from build123d import *

# Parameters (mm, degrees)
SKETCH1_R           = 8.89
SKETCH1_R_2         = 6.477
BOSS_EXTRUDE1_DEPTH = 63.5
SKETCH2_R           = 8.89
SKETCH2_R_2         = 6.477
BOSS_EXTRUDE2_DEPTH = 31.75
SKETCH4_R           = 6.477
CUT_EXTRUDE1_DEPTH  = 64.5000001
SKETCH5_R           = 6.477
CUT_EXTRUDE2_DEPTH  = 64.5000001


with BuildPart() as part:
    # Sketch1 → Boss-Extrude1 (new body)
    with BuildSketch(Plane.XY):
        Circle(SKETCH1_R)
        Circle(SKETCH1_R_2, mode=Mode.SUBTRACT)
    extrude(amount=BOSS_EXTRUDE1_DEPTH)

    # Sketch2 → Boss-Extrude2 (add, symmetric)
    with BuildSketch(Plane(origin=(0, 0, 0), x_dir=(0, 0, -1), z_dir=(1, 0, 0))):
        with Locations((-31.75, 0)):
            Circle(SKETCH2_R)
        with Locations((-31.75, 0)):
            Circle(SKETCH2_R_2, mode=Mode.SUBTRACT)
    extrude(amount=BOSS_EXTRUDE2_DEPTH, both=True)

    # Sketch4 → Cut-Extrude1 (cut, through all)
    with BuildSketch(Plane(origin=(0, 0, 0), x_dir=(-1, 0, 0), z_dir=(0, 0, -1))):
        Circle(SKETCH4_R)
    extrude(amount=-CUT_EXTRUDE1_DEPTH, mode=Mode.SUBTRACT)

    # Sketch5 → Cut-Extrude2 (cut, through all)
    with BuildSketch(Plane(origin=(31.75, 0, 0), x_dir=(0, 0, -1), z_dir=(1, 0, 0))):
        with Locations((-31.75, 0)):
            Circle(SKETCH5_R)
    extrude(amount=-CUT_EXTRUDE2_DEPTH, mode=Mode.SUBTRACT)


solid = part.part
Check sheet for the modelled part. Datum: model origin and axes. Units: mm. A direction names the side the tool comes from. Round coordinates to 2 decimals unless told otherwise and drop trailing zeros. Loops run counter-clockwise (first coordinate to the right, second up) from the corner with the lowest first, then second, coordinate; pieces in that order, holes last.
1. Sectioned sample at B-B on z = 27. Record the boundary of the cut face in (x, y), and give its area (3 significant figures).
2. Set-up check for faces 3 (the cylindrical face through (-19.18, 2.67, 23.27)), 4 (the cylindrical face through (8.212, -3.405, 12.125)), 5 (the cylindrical face through (8.48, 2.67, 50.93)): record each of +Z, -Z, +X, -X, +Y, -Y from which the full face is reachable in a straight line by a thin tool's end or side.
3. Sectioned sample at A-A on y = 0. Record the boundary of the cut face in (x, z), and give its area (3 significant figures).
4. Mould release check, pull along Y, two halves, no side actions. Record for faces 1 (the cylindrical face through (19.625, -3.405, 23.538)), 2 (the flat face through (31.75, -7, 31)): released by +Y, released by -Y, zero draft, split by the parting line, or undercut.
5. Gauge pin test, flat ends, axial feed: pin 1 Ø8 at (x, z) = (-22.5, 47.5) entering from -Y; pin 2 Ø8 at (x, z) = (-20.5, 36) entering from +Y; pin 3 Ø1 at (y, z) = (-2.5, 15) entering from +X; pin 4 Ø1.5 at (x, z) = (6.5, 36) entering from +Y. Record the tip position at first contact, or that the pin passes through.
6. Scan lines: probe 1 along Y at (x, z) = (-6, 31.75); probe 2 along Z at (x, y) = (12, 0); probe 3 along X at (y, z) = (-0.75, 4). Record each from-to range of solid material in increasing order.
7. Sectioned sample at D-D on y = -3.25. Record the boundary of the cut face in (x, z), and give its area (3 significant figures).
8. Sectioned sample at C-C on x = -20. Record the boundary of the cut face in (y, z).
Recorded:
1. outline: (-31.75, -7.51) - (-4.75, -7.51) arc R8.89 ccw to (4.75, -7.51) - (31.75, -7.51) - (31.75, -4.4) - (4.75, -4.4) arc R6.48 cw to (-4.75, -4.4) - (-31.75, -4.4) - close; (-31.75, 4.4) - (-4.75, 4.4) arc R6.48 cw to (4.75, 4.4) - (31.75, 4.4) - (31.75, 7.51) - (4.75, 7.51) arc R8.89 ccw to (-4.75, 7.51) - (-31.75, 7.51) - close
1. area: 386 mm2
2. face 3: -X
2. face 4: -Z
2. face 5: +Z
3. outline: (-31.75, 22.86) - (-8.89, 22.86) - (-8.89, 0) - (-6.48, 0) - (-6.48, 25.27) - (-31.75, 25.27) - close; (-31.75, 38.23) - (-6.48, 38.23) - (-6.48, 63.5) - (-8.89, 63.5) - (-8.89, 40.64) - (-31.75, 40.64) - close; (6.48, 0) - (8.89, 0) - (8.89, 22.86) - (31.75, 22.86) - (31.75, 25.27) - (6.48, 25.27) - close; (6.48, 38.23) - (31.75, 38.23) - (31.75, 40.64) - (8.89, 40.64) - (8.89, 63.5) - (6.48, 63.5) - close
3. area: 465 mm2
4. face 1: split by the parting line
4. face 2: zero draft
5. pin 1: passes through
5. pin 2: stops at y = 8.89
5. pin 3: stops at x = 8.66
5. pin 4: stops at y = 8.17
6. probe 1: y = -8.89 to -6.48, 6.48 to 8.89
6. probe 2: z = 22.86 to 25.27, 38.23 to 40.64
6. probe 3: x = -8.86 to -6.43, 6.43 to 8.86
7. outline: (-31.75, 23.48) - (-8.27, 23.48) - (-8.27, 0) - (-5.6, 0) - (-5.6, 26.15) - (-31.75, 26.15) - close; (-31.75, 37.35) - (-5.6, 37.35) - (-5.6, 63.5) - (-8.27, 63.5) - (-8.27, 40.02) - (-31.75, 40.02) - close; (5.6, 0) - (8.27, 0) - (8.27, 23.48) - (31.75, 23.48) - (31.75, 26.15) - (5.6, 26.15) - close; (5.6, 37.35) - (31.75, 37.35) - (31.75, 40.02) - (8.27, 40.02) - (8.27, 63.5) - (5.6, 63.5) - close
7. area: 530 mm2
8. outline: circle Ø17.78 at (0, 31.75); hole circle Ø12.95 at (0, 31.75)
